from build123d import *

# Parameters (mm, degrees)
SKETCH_10_W                = 100
SKETCH_10_H                = 130
SM_BASE_FLANGE_1_DEPTH     = 4
SKETCH_13_R                = 6
CUT_EXTRUDE_1_DEPTH        = 10
HOLE_WIZARD_M61_AT_2_COUNT = 2
HOLE_WIZARD_M61_AT_2_PITCH = 75
CHAMFER_1_SIZE             = 30
CHAMFER_1_SIZE2            = 51.961524227
FILLET_1_R                 = 34.641016
FILLET_2_R                 = 20


# Sheet-metal steps are written as plain solids
with BuildPart() as part:
    # Эскиз10 → Базовая кромка1 (new body)
    with BuildSketch(Plane(origin=(0, 0, 0), x_dir=(0, 0, -1), z_dir=(1, 0, 0))):
        with Locations((0, 65)):
            Rectangle(SKETCH_10_W, SKETCH_10_H)
    extrude(amount=-SM_BASE_FLANGE_1_DEPTH)

    # Эскиз13 → Вырез-Вытянуть1 (cut)
    with BuildSketch(Plane.ZY.offset(4)):
        with Locations((0, 110)):
            Circle(SKETCH_13_R)
    extrude(amount=-CUT_EXTRUDE_1_DEPTH, mode=Mode.SUBTRACT)

    # Эскиз16 → Зенковка для винта с потайной головкой и внутренним шестигранником M61 (revolve, cut)
    with BuildSketch(Plane(origin=(-4, 25, -37.5), x_dir=(0, 0, 1), z_dir=(0, 1, 0))):
        Polygon((0, 0), (0, 4), (3.3, 4), (3.3, 3.555), (6.855, 0), align=None)
    hole_wizard_m61 = revolve(axis=Axis((-10.35, 25, -37.5), (1, 0, 0)), mode=Mode.SUBTRACT)

    # Зенковка для винта с потайной головкой и внутренним шестигранником M61 at 2: Зенковка для винта с потайной головкой и внутренним шестигранником M61 ×2
    with Locations(*[(0, 0, i * HOLE_WIZARD_M61_AT_2_PITCH) for i in range(1, HOLE_WIZARD_M61_AT_2_COUNT)]):
        add(hole_wizard_m61, mode=Mode.SUBTRACT)

    # Фаска1
    chamfer_1_edges = [part.edges().sort_by_distance(p)[0] for p in [
        (-2, 130, 50),
        (-2, 130, -50),
    ]]
    chamfer_1_side = [part.faces().sort_by_distance(p)[0] for p in [
        (-2, 130, 0),
    ]]
    chamfer(chamfer_1_edges, length=CHAMFER_1_SIZE, length2=CHAMFER_1_SIZE2, reference=chamfer_1_side[0])

    # Скругление1
    fillet_1_edges = [part.edges().sort_by_distance(p)[0] for p in [
        (-2, 130, -20),
        (-2, 130, 20),
    ]]
    fillet(fillet_1_edges, radius=FILLET_1_R)

    # Скругление2
    fillet_2_edges = [part.edges().sort_by_distance(p)[0] for p in [
        (-2, 0, -50),
        (-2, 0, 50),
    ]]
    fillet(fillet_2_edges, radius=FILLET_2_R)


solid = part.part
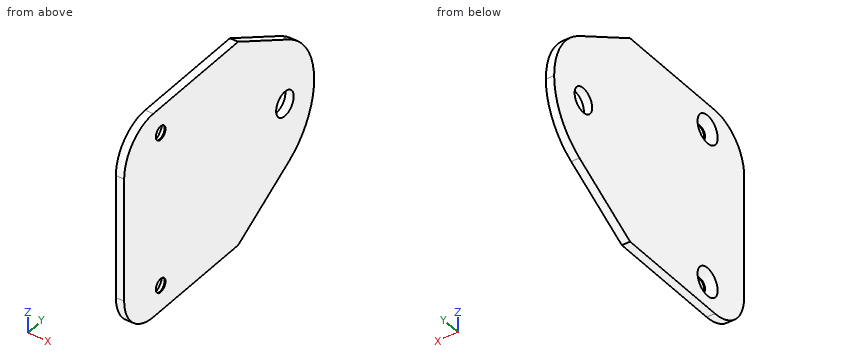
For this review, take the finished solid that the model builds, in its own axes (mm). Coordinates: 2 decimals unless noted, no trailing zeros. Order: outer loops, then holes, each group sorted by start corner. A loop starts at its lowest first (then second) coordinate and runs counter-clockwise, first axis right, second up. Notation, with made-up numbers: (84, 11) -> (137, 11) arc R13 ccw to (137, 30) -> close; hole circle Ø6 at (-16.75, 66.25). An arc over 180 degrees is marked (long way). Return JSON: item names as keys, results as strings.
1. For pin 1 Ø9.5 at (y, z) = (110, 0) entering from -X; pin 2 Ø10.5 at (y, z) = (25, -37.5) entering from -X (3 decimals), all flat-tipped, find the tip position at first contact; note any pin that passes through.
Answer block:
{"pin 1": "through", "pin 2": "x = -2.395"}
2. We need section C-C on x = -1.3. Write out the cut boundary in (y, z) (1 decimal).
Answer block:
{"outline": "(0, -30) arc R20 ccw to (20, -50) -> (78, -50) -> (112.7, -30) arc R34.6 ccw to (112.7, 30) -> (78, 50) -> (20, 50) arc R20 ccw to (0, 30) -> close; hole circle Ø8.3 at (25, -37.5); hole circle Ø8.3 at (25, 37.5); hole circle Ø12 at (110, 0)"}
3. For line 1 (Z direction, x = -0.15, y = 25); line 2 (Y direction, x = -0.3, z = -37.5); line 3 (Y direction, x = -2, z = 34), list the stretches that pass through material, from the lowest coordinate up. Write a range as from..to.
Answer block:
{"line 1": "-50..-40.8, -34.2..34.2, 40.8..50", "line 2": "1.46..21.7, 28.3..99.69", "line 3": "0.4..21.64, 28.36..105.75"}
4. We need section D-D on y = 110. Write out the cut boundary in (x, z), and give its area (3 significant figures).
Answer block:
{"outline": "(-4, -31.55) -> (0, -31.55) -> (0, -6) -> (-4, -6) -> close; (-4, 6) -> (0, 6) -> (0, 31.55) -> (-4, 31.55) -> close", "area": "204 mm²"}
5. We need section B-B on z = 37.5. Write out the cut boundary in (x, y) (1 decimal).
Answer block:
{"outline": "(-4, 1.5) -> (0, 1.5) -> (0, 21.7) -> (-0.4, 21.7) -> (-4, 18.1) -> close; (-4, 31.9) -> (-0.4, 28.3) -> (0, 28.3) -> (0, 99.7) -> (-4, 99.7) -> close"}
6. We need section A-A on y = 25. Write out the cut boundary in (x, z) (3 decimals).
Answer block:
{"outline": "(-4, -50) -> (0, -50) -> (0, -40.8) -> (-0.445, -40.8) -> (-4, -44.355) -> close; (-4, -30.645) -> (-0.445, -34.2) -> (0, -34.2) -> (0, 34.2) -> (-0.445, 34.2) -> (-4, 30.645) -> close; (-4, 44.355) -> (-0.445, 40.8) -> (0, 40.8) -> (0, 50) -> (-4, 50) -> close"}
